The listing builds one solid part. Answer for the finished solid, in the listing's coordinates (mm). Round coordinates to 2 decimals unless told otherwise and drop trailing zeros. Write each loop counter-clockwise with the first axis right and the second up, starting at its lowest first coordinate (ties: lowest second). Pieces come first, ordered by that corner, then holes.
from build123d import *

# Parameters (mm, degrees)
SKETCH_1_W      = 90.5
SKETCH_1_H      = 77
EXTRUDE_1_DEPTH = 21.6
FILLET_1_R      = 12.5


with BuildPart() as part:
    # 草圖1 → 填料-伸長1 (new body)
    with BuildSketch(Plane.XY):
        Rectangle(SKETCH_1_W, SKETCH_1_H)
    extrude(amount=EXTRUDE_1_DEPTH)

    # 圓角1
    # the kernel refuses this fillet: 12.5 mm, written as the material it takes off along each edge
    with BuildSketch(Plane(origin=(-76.5, -38.5, 0), x_dir=(0, 0, 1), z_dir=(1, 0, 0)), Plane(origin=(76.5, 38.5, 0), x_dir=(0, 0, 1), z_dir=(-1, 0, 0))) as fillet_1_piece_1:
        with BuildLine():
            CenterArc((FILLET_1_R, -FILLET_1_R), FILLET_1_R, 90, 90)
            Line((0, -FILLET_1_R), (0, 0))
            Line((0, 0), (FILLET_1_R, 0))
        make_face()
    extrude(amount=153, mode=Mode.SUBTRACT)
    with BuildSketch(Plane(origin=(-76.5, -38.5, 21.6), x_dir=(0, 0, -1), z_dir=(1, 0, 0)), Plane(origin=(76.5, 38.5, 21.6), x_dir=(0, 0, -1), z_dir=(-1, 0, 0))) as fillet_1_piece_2:
        with BuildLine():
            CenterArc((FILLET_1_R, FILLET_1_R), FILLET_1_R, 180, 90)
            Line((0, FILLET_1_R), (0, 0))
            Line((0, 0), (FILLET_1_R, 0))
        make_face()
    extrude(amount=153, mode=Mode.SUBTRACT)


solid = part.part
1. Section B-B on z = 5 is taken. Determine the outline of the cut face in (x, y).
Geometry says:
outline: (-45.25, -36) - (45.25, -36) - (45.25, 36) - (-45.25, 36) - close
2. Section C-C on z = 16.25 is taken. Determine the outline of the cut face in (x, y), plus the area to 3 significant figures.
Geometry says:
outline: (-45.25, -36.25) - (45.25, -36.25) - (45.25, 36.25) - (-45.25, 36.25) - close
area: 6,560 mm2
3. Straight lines are drawn through the part: line 1 along Z through (x, y) = (-4, 27); line 2 along Y through (x, z) = (27, 8.5); line 3 along Y through (x, z) = (31, 7). For each, find the intervals that lie inside material, in ascending order.
Geometry says:
line 1: z = 0.04 to 21.56
line 2: y = -37.84 to 37.84
line 3: y = -37.22 to 37.22
4. Given pin 1 (3 mm diameter, centred on x = -25, z = 16.5, fed in from -Y); pin 2 (2 mm diameter, centred on x = 8, z = 5, fed in from -Y); pin 3 (1 mm diameter, centred on x = -24, z = 7.5, fed in from -Y), each flat-ended and moving along its own axis, determine where each tip first touches the part or whether it passes through.
Geometry says:
pin 1: stops at y = -37.02
pin 2: stops at y = -36.68
pin 3: stops at y = -37.66
5. Section A-A on x = -6.5 is taken. Determine the outline of the cut face in (y, z).
Geometry says:
outline: (-38.38, 10.8) arc R12.5 ccw to (-26, 0) - (26, 0) arc R12.5 ccw to (38.38, 10.8) arc R12.5 ccw to (26, 21.6) - (-26, 21.6) arc R12.5 ccw to start
